Geometry: final body of the model. Coordinates: model frame, mm. Face numbers are marked on the shaded views. A direction names the side the tool comes from. Give positions to 0.01 mm unless a question says otherwise; leave off trailing zeros. Loops run counter-clockwise (first coordinate to the right, second up) from the corner with the lowest first, then second, coordinate; pieces in that order, holes last. Notation, with made-up numbers: (13.25, 68) -> (20.25, 68) arc R23 ccw to (20.25, 97) -> close; hole circle Ø7 at (42, 51). An arc over 180 degrees is marked (long way). Answer in a Markdown table with one row per item. Add a question column.
1) Draft query along Z for the marked faces 3, 4 and 5. Return one class per face: +Z half, -Z half, draft (parallel to the pull), parting line (faces both ways), or undercut.
2) Section query C-C (z = 12). Return the cut outline in (x, y), plus the area to 3 significant figures.
3) Access query for the marked faces 1 and 2. Directions: +Z, -Z, +X, -X, +Y, -Y. A direction counts if a zero-diameter tool reaches every point of the face in a straight line with its end or side. Return the directions, or none.
4) Section query D-D (y = 52). Return the cut outline in (x, z), plus the area to 3 significant figures.
5) First-contact query: P1, Ø4, axis at x = 48, z = 0, coming from the +Y side; P2, Ø12, axis at x = 48, z = -47, coming from the +Y side; P3, Ø19, axis at x = 39.5, z = -15.5, coming from the +Y side. Flat tips, straight axial feed; report the tip coordinate or a pass-through.
6) Section query B-B (y = 12.5). Return the cut outline in (x, z), plus the area to 3 significant figures.
7) Section query A-A (x = 31.5). Return the cut outline in (y, z), plus the area to 3 significant figures.
8) Line query: line 1 (Z direction, x = 59, y = 19); line 2 (X direction, y = 54, z = -53); line 3 (Y direction, x = 22.5, z = -36). Output: solid intervals per line, ascending. Write a range as from..to.
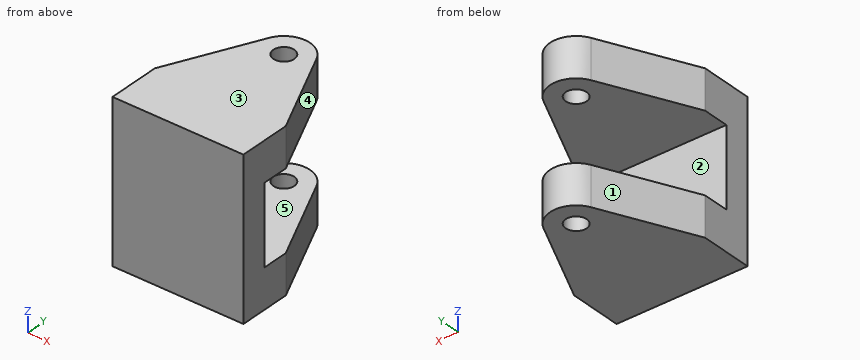
```python
from build123d import *

# Parameters (mm, degrees)
BOSS_EXTRUDE2_DEPTH = 19.05
SKETCH3_R           = 5.08
CUT_EXTRUDE1_DEPTH  = 19.05
SKETCH5_W           = 63.503429877
SKETCH5_H           = 12.7
BOSS_EXTRUDE3_DEPTH = 19.05


with BuildPart() as part:
    # Sketch2 → Boss-Extrude2 (new body)
    with BuildSketch(Plane.XY):
        with BuildLine():
            Line((2.477787128, -10.031332986), (2.477787128, 15.370038965))
            Line((2.477787128, 15.370038965), (22.715808333, 58.833279677))
            ThreePointArc((22.715808333, 58.833279677), (34.229502066, 66.172782867), (45.7431958, 58.833279677))
            Line((45.7431958, 58.833279677), (65.981217005, 15.370038965))
            Line((65.981217005, 15.370038965), (65.981217005, -10.031332986))
            Line((65.981217005, -10.031332986), (2.477787128, -10.031332986))
        make_face()
    boss_extrude2 = extrude(amount=BOSS_EXTRUDE2_DEPTH)

    # Sketch3 → Cut-Extrude1 (cut)
    with BuildSketch(Plane.XY.offset(19.05)):
        with Locations((34.229502066, 53.472096891)):
            Circle(SKETCH3_R)
    cut_extrude1 = extrude(amount=-CUT_EXTRUDE1_DEPTH, mode=Mode.SUBTRACT)

    # Sketch5 → Boss-Extrude3 (add)
    with BuildSketch(Plane(origin=(0, 0, 0), x_dir=(-1, 0, 0), z_dir=(0, 0, -1))):
        with Locations((-34.229502067, -3.681332986)):
            Rectangle(SKETCH5_W, SKETCH5_H)
    boss_extrude3 = extrude(amount=BOSS_EXTRUDE3_DEPTH)

    # Mirror1: Boss-Extrude2, Cut-Extrude1, Boss-Extrude3 across plane
    add(boss_extrude2.mirror(Plane.XY.offset(-19.05)))
    add(cut_extrude1.mirror(Plane.XY.offset(-19.05)), mode=Mode.SUBTRACT)
    add(boss_extrude3.mirror(Plane.XY.offset(-19.05)))


solid = part.part
```
Evaluation:
| question | item | result |
|---|---|---|
| 1 | face 3 | +Z half |
| 1 | face 4 | draft |
| 1 | face 5 | undercut |
| 2 | outline | (2.48, -10.03) -> (65.98, -10.03) -> (65.98, 15.37) -> (45.74, 58.83) arc R12.7 ccw to (22.72, 58.83) -> (2.48, 15.37) -> close; hole circle Ø10.16 at (34.23, 53.47) |
| 2 | area | 3,530 mm² |
| 3 | face 1 | +Z, -Z, -X, +Y |
| 3 | face 2 | +X, -X, +Y |
| 4 | outline | (19.53, -57.15) -> (29.37, -57.15) -> (29.37, -38.1) -> (19.53, -38.1) -> close; (19.53, 0) -> (29.37, 0) -> (29.37, 19.05) -> (19.53, 19.05) -> close; (39.09, -57.15) -> (48.93, -57.15) -> (48.93, -38.1) -> (39.09, -38.1) -> close; (39.09, 0) -> (48.93, 0) -> (48.93, 19.05) -> (39.09, 19.05) -> close |
| 4 | area | 749 mm² |
| 5 | P1 | y = 58.28 |
| 5 | P2 | y = 63.52 |
| 5 | P3 | y = 2.67 |
| 6 | outline | (2.48, -57.15) -> (65.98, -57.15) -> (65.98, -38.1) -> (2.48, -38.1) -> close; (2.48, 0) -> (65.98, 0) -> (65.98, 19.05) -> (2.48, 19.05) -> close |
| 6 | area | 2,420 mm² |
| 7 | outline | (-10.03, -57.15) -> (49.19, -57.15) -> (49.19, -38.1) -> (2.67, -38.1) -> (2.67, 0) -> (49.19, 0) -> (49.19, 19.05) -> (-10.03, 19.05) -> close; (57.76, -57.15) -> (65.88, -57.15) -> (65.88, -38.1) -> (57.76, -38.1) -> close; (57.76, 0) -> (65.88, 0) -> (65.88, 19.05) -> (57.76, 19.05) -> close |
| 7 | area | 3,050 mm² |
| 8 | line 1 | -57.15..-38.1, 0..19.05 |
| 8 | line 2 | 20.47..29.18, 39.28..47.99 |
| 8 | line 3 | -10.03..2.67 |
